Here's the drawing with two shaded views (mm, measured from the low corner). I have some questions. A direction names the side the tool comes from. Coordinates: 2 decimals unless noted, no trailing zeros. Order: outer loops, then holes, each group sorted by start corner. A loop starts at its lowest first (then second) coordinate and runs counter-clockwise, first axis right, second up. Notation, with made-up numbers: (-32.75, -10.5) -> (0.25, -10.5) arc R17 cw to (0.25, 11.5) -> close; hole circle Ø8 at (35, -3). An arc over 180 degrees is marked (long way). Answer as a JSON object with one key per item and string values. Group by question number.
(1) For pin 1 (2.5 mm diameter, centred on x = 37.5, z = 37, fed in from +Y); pin 2 (3 mm diameter, centred on y = 3, z = 35.5, fed in from +X) (1 decimal); pin 3 (2 mm diameter, centred on y = 12.5, z = 27, fed in from -X), each with a flat end and sliding along its axis, tell me the tip position at first contact or that it passes through.
(2) I want a section at D-D, the plane z = 36. List the corners of the cut face in (x, y) for me.
(3) I want a section at A-A, the plane x = 21. List the corners of the cut face in (y, z) for me.
(4) I want a section at C-C, the plane y = 15. List the corners of the cut face in (x, z) for me, plus the area to 3 significant figures.
(5) If we mould it in two halves opening along X, with no side actions, what happens to the marked faces 4, 5 and 6? For each: pulls with the +X half, pulls with the -X half, needs draft (parallel to the pull), parting line crosses it, or undercut.
(6) I want a section at B-B, the plane z = 21. List the corners of the cut face in (x, y) for me, plus the area to 3 significant figures.
(7) Which directions (+Z, -Z, +X, -X, +Y, -Y) give clear straight access to the entire face, cutting with the end or side of a thin tool? Please do the marked faces 1, 2 and 3.
(8) I need wall thicknesses on line 1 (Y direction, x = 37.5, z = 25.5); line 2 (Z direction, x = 24, y = 18.75); line 3 (X direction, y = 19, z = 6). Which ranges of each line are inside material? Lowest first, please.
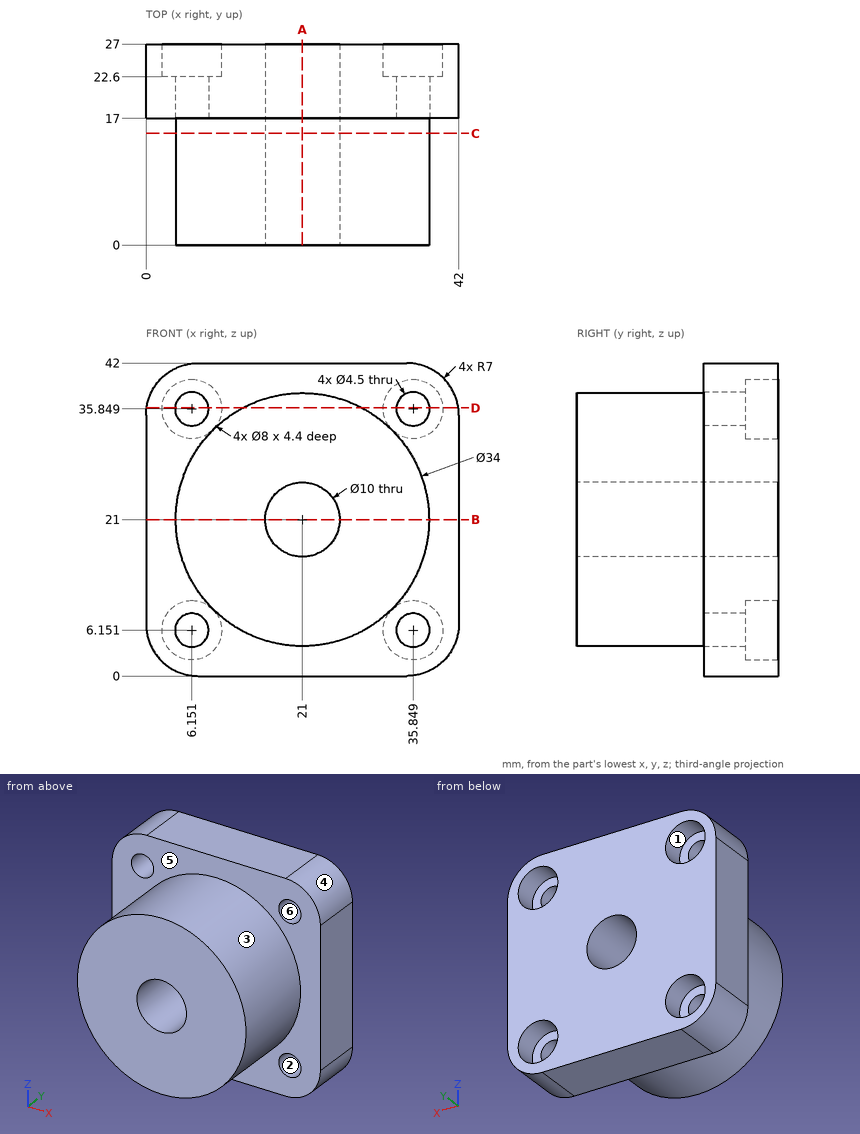
Computed values:
{
 "1": {"pin 1": "stops at y = 22.6", "pin 2": "stops at x = 32", "pin 3": "stops at x = 4.75"},
 "2": {"outline": "(0.07, 17) -> (3.91, 17) -> (3.91, 22.6) -> (2.15, 22.6) -> (2.15, 27) -> (0.07, 27) -> close; (8.4, 17) -> (13, 17) -> (13, 0) -> (29, 0) -> (29, 17) -> (33.6, 17) -> (33.6, 22.6) -> (31.85, 22.6) -> (31.85, 27) -> (10.15, 27) -> (10.15, 22.6) -> (8.4, 22.6) -> close; (38.09, 17) -> (41.93, 17) -> (41.93, 27) -> (39.85, 27) -> (39.85, 22.6) -> (38.09, 22.6) -> close"},
 "3": {"outline": "(0, 4) -> (17, 4) -> (17, 0) -> (27, 0) -> (27, 16) -> (0, 16) -> close; (0, 26) -> (27, 26) -> (27, 42) -> (17, 42) -> (17, 38) -> (0, 38) -> close"},
 "4": {"outline": "circle Ø34 at (21, 21); hole circle Ø10 at (21, 21)", "area": "829 mm2"},
 "5": {"face 4": "pulls with the +X half", "face 5": "needs draft", "face 6": "undercut"},
 "6": {"outline": "(0, 17) -> (4, 17) -> (4, 0) -> (16, 0) -> (16, 27) -> (0, 27) -> close; (26, 0) -> (38, 0) -> (38, 17) -> (42, 17) -> (42, 27) -> (26, 27) -> close", "area": "728 mm2"},
 "7": {"face 1": "+Y", "face 2": "+Y, -Y", "face 3": "-Y"},
 "8": {"line 1": "y = 17 to 27", "line 2": "z = 0 to 17, 25 to 42", "line 3": "x = 0.07 to 3.91, 8.4 to 33.6, 38.09 to 41.93"}
}
